```python
from build123d import *

# Parameters (mm, degrees)
BOSS_EXTRUDE1_DEPTH   = 105
BOSS_EXTRUDE1_2_DEPTH = 105
BOSS_EXTRUDE6_DEPTH   = 15
BOSS_EXTRUDE9_START   = -30
BOSS_EXTRUDE9_DEPTH   = 30
BOSS_EXTRUDE10_DEPTH  = 30
SKETCH7_W             = 350
SKETCH7_H             = 200
BOSS_EXTRUDE11_DEPTH  = 20
SKETCH8_W             = 350
SKETCH8_H             = 200
BOSS_EXTRUDE12_DEPTH  = 20
SKETCH9_R             = 20
CUT_EXTRUDE1_DEPTH    = 300
SKETCH10_R            = 5
CUT_EXTRUDE2_DEPTH    = 20


with BuildPart() as part:
    # Sketch1 → Boss-Extrude1 (new, symmetric)
    with BuildSketch(Plane.XY):
        with BuildLine():
            Line((125, -35.707142143), (125, -54.024352148))
            ThreePointArc((125, -54.024352148), (118.230654865, -67.565841039), (110, -80.27222823))
            Line((110, -80.27222823), (110, -200))
            Line((110, -200), (125, -200))
            Line((125, -200), (175, -200))
            Line((175, -200), (175, 0))
            Line((175, 0), (125, 0))
            ThreePointArc((125, 0), (121.191996435, -30.618621785), (110, -59.371710435))
            Line((110, -59.371710435), (110, -69.282032303))
            ThreePointArc((110, -69.282032303), (118.693168769, -53.027650218), (125, -35.707142143))
        make_face()
    extrude(amount=BOSS_EXTRUDE1_DEPTH, both=True)



with BuildPart() as body_2:
    # Sketch1 → Boss-Extrude1 2 (new, symmetric)
    with BuildSketch(Plane.XY):
        with BuildLine():
            Line((-110, -200), (-125, -200))
            Line((-125, -200), (-175, -200))
            Line((-175, -200), (-175, 0))
            Line((-175, 0), (-125, 0))
            ThreePointArc((-125, 0), (-121.191996435, -30.618621785), (-110, -59.371710435))
            Line((-110, -59.371710435), (-110, -69.282032303))
            ThreePointArc((-110, -69.282032303), (-118.693168769, -53.027650218), (-125, -35.707142143))
            Line((-125, -35.707142143), (-125, -54.024352148))
            ThreePointArc((-125, -54.024352148), (-118.230654865, -67.565841039), (-110, -80.27222823))
            Line((-110, -80.27222823), (-110, -200))
        make_face()
    extrude(amount=BOSS_EXTRUDE1_2_DEPTH, both=True)


with BuildPart() as part_1:
    add(part.part)

    add(body_2.part)  # Boss-Extrude6 merges body 2
    # Sketch6 → Boss-Extrude6 (add, symmetric)
    with BuildSketch(Plane.XY):
        with BuildLine():
            Line((-110, -69.282032303), (-110, -59.371710435))
            ThreePointArc((-110, -59.371710435), (-121.191996435, -30.618621785), (-125, 0))
            Line((-125, 0), (125, 0))
            ThreePointArc((125, 0), (121.191996435, -30.618621785), (110, -59.371710435))
            Line((110, -59.371710435), (110, -69.282032303))
            Line((110, -69.282032303), (-110, -69.282032303))
        make_face()
    extrude(amount=BOSS_EXTRUDE6_DEPTH, both=True)

    # 3DSketch3 → Boss-Extrude9 (add)
    with BuildSketch(Plane(origin=(-110, -59.371710435, 45), x_dir=(0.9695359714832644, 0.2449489742783234, 0), z_dir=(0, 0, -1)).offset(BOSS_EXTRUDE9_START)):
        with BuildLine():
            Line((0, 0), (-2.427523176, 9.60841354))
            Line((-2.427523176, 9.60841354), (210.87039055, 63.497187881))
            Line((210.87039055, 63.497187881), (213.297913726, 53.888774341))
            ThreePointArc((213.297913726, 53.888774341), (231.191996435, 28.75308865), (242.383992871, 0))
            Line((242.383992871, 0), (0, -61.23724357))
            ThreePointArc((0, -61.23724357), (-3.808003565, -30.618621785), (0, 0))
        make_face()
    extrude(amount=BOSS_EXTRUDE9_DEPTH)

    # 3DSketch4 → Boss-Extrude10 (add)
    with BuildSketch(Plane(origin=(110, -59.371710435, -45), x_dir=(-0.9695359714832668, 0.2449489742783143, 0), z_dir=(0, 0, 1))):
        with BuildLine():
            Line((0, 0), (-2.427523176, 9.60841354))
            Line((-2.427523176, 9.60841354), (210.87039055, 63.497187881))
            Line((210.87039055, 63.497187881), (213.297913726, 53.888774341))
            ThreePointArc((213.297913726, 53.888774341), (231.191996435, 28.75308865), (242.383992871, 0))
            Line((242.383992871, 0), (0, -61.23724357))
            ThreePointArc((0, -61.23724357), (-3.808003565, -30.618621785), (0, 0))
        make_face()
    extrude(amount=-BOSS_EXTRUDE10_DEPTH)

    # Sketch7 → Boss-Extrude11 (add)
    with BuildSketch(Plane.XY.offset(105)):
        with Locations((0, -100)):
            Rectangle(SKETCH7_W, SKETCH7_H)
    extrude(amount=BOSS_EXTRUDE11_DEPTH)

    # Sketch8 → Boss-Extrude12 (add)
    with BuildSketch(Plane(origin=(0, 0, -105), x_dir=(-1, 0, 0), z_dir=(0, 0, -1))):
        with Locations((0, -100)):
            Rectangle(SKETCH8_W, SKETCH8_H)
    extrude(amount=BOSS_EXTRUDE12_DEPTH)

    # Sketch9 → Cut-Extrude1 (cut)
    with BuildSketch(Plane.XY.offset(125)):
        Circle(SKETCH9_R)
    extrude(amount=-CUT_EXTRUDE1_DEPTH, mode=Mode.SUBTRACT)

    # Sketch10 → Cut-Extrude2 (cut)
    with BuildSketch(Plane(origin=(0, 0, 0), x_dir=(1, 0, 0), z_dir=(0, 1, 0))):
        with Locations(Location((150, 50, 0), (0, 0, 270))):
            Circle(SKETCH10_R)
        with Locations(Location((150, -50, 0), (0, 0, 90))):
            Circle(SKETCH10_R)
        with Locations(Location((-150, -50, 0), (0, 0, 270))):
            Circle(SKETCH10_R)
        with Locations(Location((-150, 50, 0), (0, 0, 90))):
            Circle(SKETCH10_R)
    extrude(amount=-CUT_EXTRUDE2_DEPTH, mode=Mode.SUBTRACT)


solid = part_1.part
```
Source: CAD feature listing. Evaluate the final solid. Frame: model axes, mm. A direction names the side the tool comes from. Round coordinates to 2 decimals unless told otherwise and drop trailing zeros. Loops run counter-clockwise (first coordinate to the right, second up) from the corner with the lowest first, then second, coordinate; pieces in that order, holes last. Notation, with made-up numbers: M 46,-3 L 61,-3 A19 cw 61,11 Z; hole C 23,6.25 d8. An arc over 180 degrees is marked long. Put each result on its own line as item: value.
(1) Section C-C, the plane y = -63.5. Return loops of the section in (x, z).
Solutions:
outline: M -175,-125 L 175,-125 L 175,125 L -175,125 Z; hole M -120.46,-105 L -113.44,-105 L -113.44,105 L -120.46,105 Z; hole M -110,-105 L 110,-105 L 110,-75 L -110,-75 Z; hole M -110,-45 L 110,-45 L 110,-15 L -110,-15 Z; hole M -110,15 L 110,15 L 110,45 L -110,45 Z; hole M -110,75 L 110,75 L 110,105 L -110,105 Z; hole M 113.44,-105 L 120.46,-105 L 120.46,105 L 113.44,105 Z
(2) Pull-direction query (Z, two-part tool) for faces 1 (the face through (2, -99, -125)), 2 (the face through (-121.297, -30.199, -89.79)), 3 (the face through (-154.88, -9.86, 48.92)), 4 (the face through (0, -20, 60)); classes: released by +Z, released by -Z, zero draft, split by the parting line, or undercut.
Solutions:
face 1: released by -Z
face 2: undercut
face 3: undercut
face 4: zero draft
(3) Section D-D, the plane z = -4. Return loops of the section in (x, y) (3 decimals).
Solutions:
outline: M -175,-200 L -110,-200 L -110,-80.272 A136.175 cw -125,-54.024 L -125,-35.707 A130 ccw -110,-69.282 L 110,-69.282 A130 ccw 125,-35.707 L 125,-54.024 A136.175 cw 110,-80.272 L 110,-200 L 175,-200 L 175,0 L 20,0 A20 cw -20,0 L -175,0 Z
(4) Ray query, line 1 (X direction, y = -7, z = -50) (3 decimals); line 2 (X direction, y = -163, z = 84); line 3 (Z direction, x = 25, y = -20). Return the intervals inside material, ascending. Write a range as [from, to].
Solutions:
line 1: [-175, -155], [-145, -18.735], [18.735, 145], [155, 175]
line 2: [-175, -110], [110, 175]
line 3: [-125, -105], [-75, -45], [-15, 15], [45, 75], [105, 125]
(5) Access query for faces 5 (the face through (110, -64, 30)), 6 (the face through (-118.336, -67.382, 1.47)), 7 (the face through (110, -139, 1)), 8 (the face through (-121.297, -30.199, -29.79)), 9 (the face through (0, -20, 115)). Directions: +Z, -Z, +X, -X, +Y, -Y. A direction counts if a zero-diameter tool reaches every point of the face in a straight line with its end or side. Return the directions, or none.
Solutions:
face 5: +Y, -Y
face 6: none
face 7: -Y
face 8: +Y
face 9: +Z, -Z, +Y
(6) First-contact query: pin 1 (8 mm diameter, centred on x = 148.5, z = -52, fed in from +Y); pin 2 (8 mm diameter, centred on x = -150, z = 50, fed in from +Y); pin 3 (10 mm diameter, centred on x = -32.5, z = 13.5, fed in from -Y). Flat tips, straight axial feed; report the tip coordinate or a pass-through.
Solutions:
pin 1: y = 0
pin 2: y = -20
pin 3: y = -69.28
(7) Section B-B, the plane z = 31. Return loops of the section in (x, y) (3 decimals), and give its area (3 significant figures).
Solutions:
outline: M -175,-200 L -110,-200 L -110,-80.272 A136.175 cw -125,-54.024 L -125,-35.707 A130 ccw -110,-69.282 L -110,-59.372 A125 cw -125,0 L -175,0 Z; M 110,-200 L 175,-200 L 175,0 L 125,0 A125 cw 110,-59.372 L 110,-69.282 A130 ccw 125,-35.707 L 125,-54.024 A136.175 cw 110,-80.272 Z
area: 24,400 mm²
(8) Section A-A, the plane x = -54.5. Return loops of the section in (y, z), and give its area (3 significant figures).
Solutions:
outline: M -200,-125 L 0,-125 L 0,-105 L -200,-105 Z; M -200,105 L 0,105 L 0,125 L -200,125 Z; M -69.28,-75 L 0,-75 L 0,-45 L -69.28,-45 Z; M -69.28,-15 L 0,-15 L 0,15 L -69.28,15 Z; M -69.28,45 L 0,45 L 0,75 L -69.28,75 Z
area: 14,200 mm²
